from build123d import *

# Parameters (mm, degrees)
SKETCH_1_W                   = 50
SKETCH_1_H                   = 68
EXTRUDE_1_DEPTH              = 8
SKETCH_2_R                   = 2
CUT_EXTRUDE_1_DEPTH          = 43.95346319
HOLE_WIZARD_M4_1_D           = 3.3
HOLE_WIZARD_M4_1_DEPTH       = 10.1
HOLE_WIZARD_M4_1_CSINK_D     = 4.05
HOLE_WIZARD_M4_1_CSINK_ANGLE = 90
HOLE_WIZARD_M4_1_TIP         = 0.991420021
MM_1_D                       = 3
MM_1_DEPTH                   = 8
MM_1_TIP                     = 0.901290929
FILLET_1_R                   = 10
FILLET_2_R                   = 1


with BuildPart() as part:
    # 草图1 → 凸台-拉伸1 (new body)
    with BuildSketch(Plane.XY):
        Rectangle(SKETCH_1_W, SKETCH_1_H)
    extrude(amount=EXTRUDE_1_DEPTH)

    # 草图2 → 切除-拉伸1 (cut, through all)
    with BuildSketch(Plane.XY.offset(8)):
        with Locations((-11.5, -16)):
            Circle(SKETCH_2_R)
        with Locations((-11.5, 24)):
            Circle(SKETCH_2_R)
        with Locations(Location((11.5, 24, 0), (0, 0, 180))):
            Circle(SKETCH_2_R)
        with Locations(Location((11.5, -16, 0), (0, 0, 180))):
            Circle(SKETCH_2_R)
    extrude(amount=-CUT_EXTRUDE_1_DEPTH, mode=Mode.SUBTRACT)

    # M4 螺纹孔1
    with Locations(Plane(origin=(-20, -34, 4), x_dir=(0, 0, -1), z_dir=(0, -1, 0))):
        with Locations((0, 0), (0, 40)):
            CounterSinkHole(HOLE_WIZARD_M4_1_D / 2, HOLE_WIZARD_M4_1_CSINK_D / 2, depth=HOLE_WIZARD_M4_1_DEPTH, counter_sink_angle=HOLE_WIZARD_M4_1_CSINK_ANGLE)
            with Locations((0, 0, -(HOLE_WIZARD_M4_1_DEPTH + HOLE_WIZARD_M4_1_TIP / 2))):  # 118° drill point
                Cone(0, HOLE_WIZARD_M4_1_D / 2, HOLE_WIZARD_M4_1_TIP, mode=Mode.SUBTRACT)

    # 大小mm 暗销孔1
    with Locations(Plane(origin=(-12.5, -34, 4), x_dir=(0, 0, -1), z_dir=(0, -1, 0))):
        with Locations((0, 0), (0, 25)):
            Hole(MM_1_D / 2, depth=MM_1_DEPTH)
            with Locations((0, 0, -(MM_1_DEPTH + MM_1_TIP / 2))):  # 118° drill point
                Cone(0, MM_1_D / 2, MM_1_TIP, mode=Mode.SUBTRACT)

    # 圆角1
    fillet_1_edges = [part.edges().sort_by_distance(p)[0] for p in [
        (-25, 34, 4),
        (25, 34, 4),
    ]]
    fillet(fillet_1_edges, radius=FILLET_1_R)

    # 圆角2
    fillet_2_edges = [part.edges().sort_by_distance(p)[0] for p in [
        (25, -34, 4),
        (-25, -34, 4),
    ]]
    fillet(fillet_2_edges, radius=FILLET_2_R)


solid = part.part
The listing builds one solid part. Answer for the finished solid, in the listing's coordinates (mm). A direction names the side the tool comes from. Give positions to 0.01 mm unless a question says otherwise; leave off trailing zeros. Order: outer loops, then holes, each group sorted by start corner. A loop starts at its lowest first (then second) coordinate and runs counter-clockwise, first axis right, second up. Notation, with made-up numbers: (69, 69) -> (96, 69) arc R15 cw to (96, 97) -> close; hole circle Ø3 at (-4.75, 48). An arc over 180 degrees is marked (long way). Put each result on its own line as item: value.
Item 1: For faces 1 (the face through (-13.075, -29.944, 5.386)), 2 (the face through (25, -5, 4)), determine the directions among +Z, -Z, +X, -X, +Y, -Y from which every point of the face is accessible in a straight line to the end or side of a thin tool.
Established:
face 1: -Y
face 2: +Z, -Z, +X, +Y, -Y
Item 2: A cutting plane is placed at B-B on y = 25. Give the vertices of the cut face in (x, z), plus the area to 3 significant figures.
Established:
outline: (-24.95, 0) -> (-13.23, 0) -> (-13.23, 8) -> (-24.95, 8) -> close; (-9.77, 0) -> (9.77, 0) -> (9.77, 8) -> (-9.77, 8) -> close; (13.23, 0) -> (24.95, 0) -> (24.95, 8) -> (13.23, 8) -> close
area: 344 mm^2
Item 3: Given P1, Ø2.5, axis at x = 20, z = 4, coming from the +Y side; P2, Ø3, axis at x = -20, z = 4, coming from the -Y side, each flat-ended and moving along its own axis, determine where each tip first touches the part or whether it passes through.
Established:
P1: stops at y = 33.27
P2: stops at y = -23.81
Item 4: Straight lines are drawn through the part: line 1 (X direction, y = -29.25, z = 4); line 2 (X direction, y = -28, z = 3); line 3 (Y direction, x = 10, z = 5). For each, find the intervals that lie inside material, in ascending order.
Established:
line 1: x = -25 to -21.65, -18.35 to -14, -11 to 11, 14 to 18.35, 21.65 to 25
line 2: x = -25 to -21.31, -18.69 to -13.62, -11.38 to 11.38, 13.62 to 18.69, 21.31 to 25
line 3: y = -34 to -17.32, -14.68 to 22.68, 25.32 to 34
Item 5: A cutting plane is placed at A-A on z = 7.25. Give the vertices of the cut face in (x, y).
Established:
outline: (-25, -33) arc R1 ccw to (-24, -34) -> (24, -34) arc R1 ccw to (25, -33) -> (25, 24) arc R10 ccw to (15, 34) -> (-15, 34) arc R10 ccw to (-25, 24) -> close; hole circle Ø4 at (-11.5, -16); hole circle Ø4 at (-11.5, 24); hole circle Ø4 at (11.5, -16); hole circle Ø4 at (11.5, 24)
Item 6: For a pull along Z with two mould halves and no side action, classify faces 3 (the face through (21.99, 31.15, 4.06)), 4 (the face through (12.269, -25.255, 3.88)), 5 (the face through (0, 0, 8)) as released by +Z, released by -Z, zero draft, split by the parting line, or undercut.
Established:
face 3: zero draft
face 4: undercut
face 5: released by +Z
